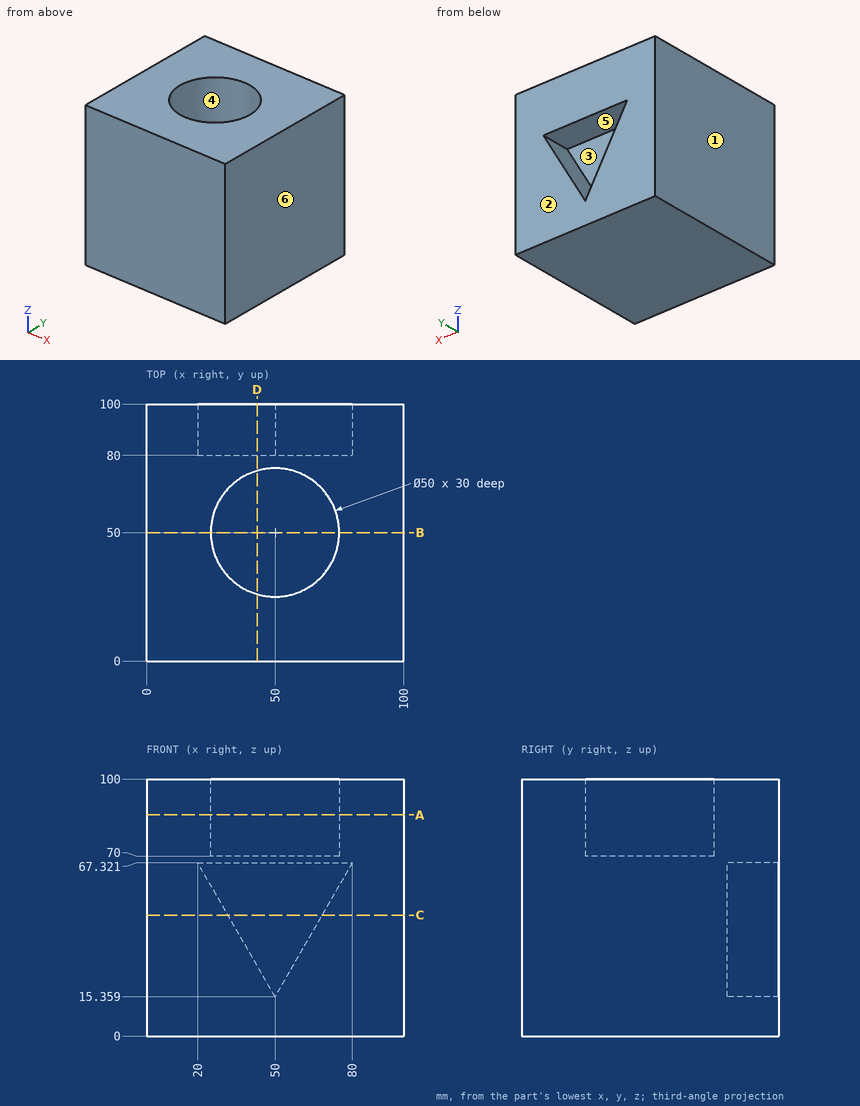
Check sheet for the drawn part. Datum: minimum x, y, z corner. Units: mm. A direction names the side the tool comes from. Round coordinates to 2 decimals unless told otherwise and drop trailing zeros. Write each loop counter-clockwise with the first axis right and the second up, starting at its lowest first coordinate (ties: lowest second). Pieces come first, ordered by that corner, then holes. Notation, with made-up numbers: (-32, -29) - (-17, -29) arc R15 ccw to (-17, -22) - close; hole circle Ø1 at (21.25, 55.25). An arc over 180 degrees is marked (long way). Write each question's results on one line, items separated by ' | '.
(1) Sectioned sample at B-B, the plane y = 50. Enter the section's corners in (x, z).
Computed:
outline: (0, 0) - (100, 0) - (100, 100) - (75, 100) - (75, 70) - (25, 70) - (25, 100) - (0, 100) - close
(2) Draft check along X on the marked faces 1, 2 and 3. Enter one of: pulls with the +X half, pulls with the -X half, needs draft (parallel to the pull), parting line crosses it, or undercut.
Computed:
face 1: pulls with the -X half | face 2: needs draft | face 3: undercut
(3) Thickness scan on probe 1 along Y at (x, z) = (50, 86); probe 2 along X at (y, z) = (51, 95); probe 3 along Z at (x, y) = (36.5, 51). Record the ranges inside material, lowest first. Write a range as from..to.
Computed:
probe 1: y = 0..25, 75..100 | probe 2: x = 0..25.02, 74.98..100 | probe 3: z = 0..70
(4) Sectioned sample at C-C, the plane z = 47. Enter the section's corners in (x, y).
Computed:
outline: (0, 0) - (100, 0) - (100, 100) - (68.27, 100) - (68.27, 80) - (31.73, 80) - (31.73, 100) - (0, 100) - close
(5) Sectioned sample at A-A, the plane z = 86. Enter the section's corners in (x, y).
Computed:
outline: (0, 0) - (100, 0) - (100, 100) - (0, 100) - close; hole circle Ø50 at (50, 50)
(6) Set-up check for the marked faces 4, 5 and 6: record each of +Z, -Z, +X, -X, +Y, -Y from which the full face is reachable in a straight line by a thin tool's end or side.
Computed:
face 4: +Z | face 5: +Y | face 6: +Z, -Z, +X, +Y, -Y
(7) Sectioned sample at D-D, the plane x = 43. Enter the section's corners in (y, z), plus the area to 3 significant figures.
Computed:
outline: (0, 0) - (100, 0) - (100, 27.48) - (80, 27.48) - (80, 67.32) - (100, 67.32) - (100, 100) - (74, 100) - (74, 70) - (26, 70) - (26, 100) - (0, 100) - close | area: 7,760 mm^2
